```python
from build123d import *

# Parameters (mm, degrees)
F0_W         = 40
F0_H         = 20
F1_DEPTH     = 40
F2_R         = 9
F3_DEPTH     = 74.7
F4_R         = 8
F5_T1_DEPTH  = 40
F5_T4_ANGLE  = 90
F5_T6_ANGLE  = 90
F5_T8_ANGLE  = 90
F5_T10_ANGLE = 90


# Not quite as in the source:
# - a fillet or chamfer that OpenCascade refuses, or shapes differently, is made with other operations: its cross-section is extruded or revolved along the edge and cut away or added
# - a pattern or mirror of a feature is missing from the dataset's text; its kind, count and spacing are read off the source's solid


with BuildPart() as f1:
    # F0 (on Front) → F1 (new body)
    with BuildSketch(Plane.XZ):
        Polygon((-120, 20), (-120, 0), (-90, 0), (-90, 52), (0, 52), (90, 52), (90, 0), (120, 0), (160, 0), (160, 20), (120, 20), (120, 52), (120, 77), (0, 77), (-120, 77), (-120, 52), align=None)
        with Locations((-140, 10)):
            Rectangle(F0_W, F0_H)
    extrude(amount=F1_DEPTH)

    # F2 (on face) → F3 (cut)
    with BuildSketch(Plane.XY.offset(20)):
        with Locations((-140, -20)):
            Circle(F2_R)
    f3 = extrude(amount=-F3_DEPTH, mode=Mode.SUBTRACT)

    # F3_copies: F3 across plane
    add(f3.mirror(Plane(origin=(0, 0, 0), x_dir=(0, 0, 1), z_dir=(1, 0, 0))), mode=Mode.SUBTRACT)

    # F4
    f4_edges = [f1.edges().sort_by_distance(p)[0] for p in [
        (-160, -40, 10),
        (-160, 0, 10),
        (160, 0, 10),
        (160, -40, 10),
        (140, 0, 20),
        (120, 0, 48.5),
        (0, 0, 77),
        (-120, 0, 48.5),
        (-140, 0, 20),
        (-140, -40, 20),
        (-120, -40, 48.5),
        (0, -40, 77),
        (120, -40, 48.5),
        (140, -40, 20),
        (160, -20, 20),
        (160, -20, 0),
        (90, 0, 26),
        (0, 0, 52),
        (-90, 0, 26),
        (-125, 0, 0),
        (-160, -20, 0),
        (-125, -40, 0),
        (-90, -40, 26),
        (0, -40, 52),
        (90, -40, 26),
        (125, -40, 0),
        (90, -20, 0),
        (90, -20, 52),
        (-90, -20, 52),
        (-160, -20, 20),
        (125, 0, 0),
        (-90, -20, 0),
    ]]
    fillet(f4_edges, radius=F4_R)

    # F5: fillet of radius 35 on 2 edges, made by hand

    # F5_s2 → F5_t1 (cut)
    with BuildSketch(Plane.XZ):
        with BuildLine():
            ThreePointArc((-120, 42), (-109.7487373415, 66.7487373415), (-85, 77))
            Line((-85, 77), (-120, 77))
            Line((-120, 77), (-120, 42))
        make_face()
        with BuildLine():
            ThreePointArc((85, 77), (109.7487373415, 66.7487373415), (120, 42))
            Line((120, 42), (120, 77))
            Line((120, 77), (85, 77))
        make_face()
    extrude(amount=F5_T1_DEPTH, mode=Mode.SUBTRACT)

    # F5_s3 → F5_t4 (revolve, cut)
    with BuildSketch(Plane.YZ.offset(85)):
        with BuildLine():
            ThreePointArc((0, 69), (-2.3431457505, 74.6568542495), (-8, 77))
            Line((-8, 77), (0, 77))
            Line((0, 77), (0, 69))
        make_face()
    revolve(axis=Axis((85, 0, 42), (0, 1, 0)), revolution_arc=F5_T4_ANGLE, mode=Mode.SUBTRACT)

    # F5_s5 → F5_t6 (revolve, cut)
    with BuildSketch(Plane.XY.offset(42)):
        with BuildLine():
            ThreePointArc((112, -40), (117.6568542495, -37.6568542495), (120, -32))
            Line((120, -32), (120, -40))
            Line((120, -40), (112, -40))
        make_face()
    revolve(axis=Axis((85, -40, 42), (0, -1, 0)), revolution_arc=F5_T6_ANGLE, mode=Mode.SUBTRACT)

    # F5_s7 → F5_t8 (revolve, cut)
    with BuildSketch(Plane.XY.offset(42)):
        with BuildLine():
            ThreePointArc((-112, 0), (-117.6568542495, -2.3431457505), (-120, -8))
            Line((-120, -8), (-120, 0))
            Line((-120, 0), (-112, 0))
        make_face()
    revolve(axis=Axis((-85, 0, 42), (0, 1, 0)), revolution_arc=F5_T8_ANGLE, mode=Mode.SUBTRACT)

    # F5_s9 → F5_t10 (revolve, cut)
    with BuildSketch(Plane.YZ.offset(-85)):
        with BuildLine():
            ThreePointArc((-40, 69), (-37.6568542495, 74.6568542495), (-32, 77))
            Line((-32, 77), (-40, 77))
            Line((-40, 77), (-40, 69))
        make_face()
    revolve(axis=Axis((-85, -40, 42), (0, -1, 0)), revolution_arc=F5_T10_ANGLE, mode=Mode.SUBTRACT)


solid = f1.part
```
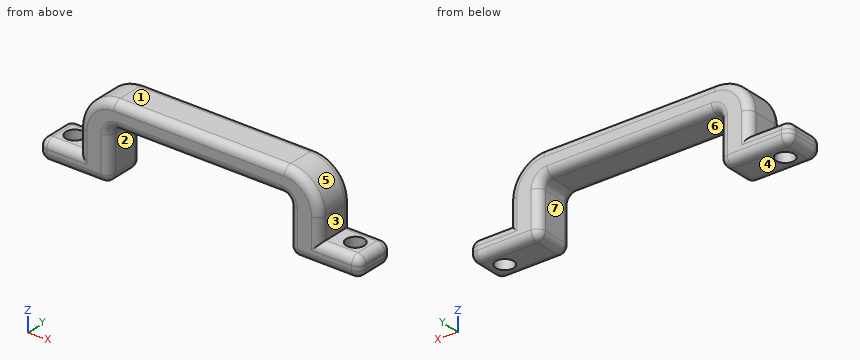
Verification items for the finished model (mm, model axes). Face numbers are marked on the shaded views. A direction names the side the tool comes from. Coordinates: 2 decimals unless noted, no trailing zeros. Order: outer loops, then holes, each group sorted by start corner. A loop starts at its lowest first (then second) coordinate and runs counter-clockwise, first axis right, second up. Notation, with made-up numbers: (-2, 80) -> (55, 80) arc R14 cw to (55, 105) -> close; hole circle Ø10 at (62, 1.5). An arc over 180 degrees is marked (long way). Put each result on its own line as item: value. Start each with the question number.
1) Cross-section at B-B (x = 140). Enter the section's corners in (y, z), plus the area to 3 significant figures.
2) Material ranges on L1, parallel to Y at x = -140, z = 11.25; L2, parallel to X at y = -32.5, z = 30.5; L3, parallel to Z at x = 53, y = -22.5, recorded low to high.
3) Cross-section at D-D (y = -5). Enter the section's corners in (x, z).
4) Cross-section at A-A (y = -20). State how many separate pieces and enclosed holes the cut face has, plus the area to 3 significant figures.
5) Release check for a two-part mould opening along X. For the marked faces 4, 5, 6 and 7 record: pulls with the +X half, pulls with the -X half, needs draft (parallel to the pull), parting line crosses it, or undercut.
6) Go/stop test with flat-tipped pins: pin 1 (3 mm diameter, centred on x = -101.5, z = 68.5, fed in from -Y); pin 2 (7 mm diameter, centred on y = -19, z = 24.5, fed in from -X); pin 3 (17.5 mm diameter, centred on y = -26, z = 29.5, fed in from +X); pin 4 (2 mm diameter, centred on x = 44, y = -33, fed in from +Z). Record where each tip stops, or that it passes through.
7) Cross-section at C-C (x = 68.5). Enter the section's corners in (y, z).
8) Tool access check on the marked faces 1, 2 and 3. Record the directions out of +Z, -Z, +X, -X, +Y, -Y that give a thin tool (end or side, any length) a straight path to the whole face; none if there is none.
Geometry check:
1. outline: (-40, 8) arc R8 ccw to (-32, 0) -> (-29, 0) -> (-29, 20) -> (-32, 20) arc R8 ccw to (-40, 12) -> close; (-11, 0) -> (-8, 0) arc R8 ccw to (0, 8) -> (0, 12) arc R8 ccw to (-8, 20) -> (-11, 20) -> close
1. area: 385 mm^2
2. L1: y = -40 to -29, -11 to 0
2. L2: x = -119.98 to -90.02, 90.02 to 119.98
2. L3: z = 52 to 77
3. outline: (-159.42, 8) arc R7.42 ccw to (-152, 0.58) -> (-98, 0.58) arc R7.42 ccw to (-90.58, 8) -> (-90.58, 44) arc R8.58 cw to (-82, 52.58) -> (82, 52.58) arc R8.58 cw to (90.58, 44) -> (90.58, 8) arc R7.42 ccw to (98, 0.58) -> (152, 0.58) arc R7.42 ccw to (159.42, 8) -> (159.42, 12) arc R7.42 ccw to (152, 19.42) -> (119.42, 19.42) -> (119.42, 42) arc R34.42 ccw to (85, 76.42) -> (-85, 76.42) arc R34.42 ccw to (-119.42, 42) -> (-119.42, 19.42) -> (-152, 19.42) arc R7.42 ccw to (-159.42, 12) -> close
4. separate pieces: 3
4. enclosed holes: 0
4. area: 9,420 mm^2
5. face 4: needs draft
5. face 5: pulls with the +X half
5. face 6: undercut
5. face 7: undercut
6. pin 1: stops at y = -39.52
6. pin 2: stops at x = -120
6. pin 3: stops at x = 120
6. pin 4: stops at z = 77
7. outline: (-40, 60) arc R8 ccw to (-32, 52) -> (-8, 52) arc R8 ccw to (0, 60) -> (0, 69) arc R8 ccw to (-8, 77) -> (-32, 77) arc R8 ccw to (-40, 69) -> close
8. face 1: +Z, +X, -X, +Y, -Y
8. face 2: -Z, +Y, -Y
8. face 3: +Z, +X, +Y, -Y
